Geometry check sheet. Reference: the model listing, model coordinates, mm. A direction names the side the tool comes from. Round coordinates to 2 decimals unless told otherwise and drop trailing zeros. Order: outer loops, then holes, each group sorted by start corner. A loop starts at its lowest first (then second) coordinate and runs counter-clockwise, first axis right, second up. Notation, with made-up numbers: (18, 58) - (32, 58) arc R21 ccw to (32, 75) - close; hole circle Ø10 at (21, 38). An arc over 180 degrees is marked (long way). One line per question, with ' | ' between items. Start each with the question number.
Q1. Sectioned sample at B-B, the plane z = -2. Give the number of separate pieces and of enclosed holes in the cut face, then the cut area to 3 significant figures.
Q2. Mould release check, pull along X, two halves, no side actions. Record for faces 3 (the face through (1, 12, -1)), 4 (the face through (-70.935, -5, -1)), 5 (the face through (41.515, 1.481, -1.369)): +X half, -X half, draft (parallel to the pull), parting line (faces both ways), or undercut.
Q3. Sectioned sample at C-C, the plane y = -5. Enter the section's corners in (x, z) (1 decimal), then the cut area to 3 significant figures.
Q4. Sectioned sample at A-A, the plane y = 1. Enter the section's corners in (x, z) (1 decimal), then the cut area to 3 significant figures.
Q5. Tool access check on faces 1 (the face through (-1, -23, -1)), 2 (the face through (63, 4, -1)). Record the directions out of +Z, -Z, +X, -X, +Y, -Y that give a thin tool (end or side, any length) a straight path to the whole face; none if there is none.
Q6. Material ranges on line 1 along X through (y, z) = (-4, -1.65) (1 decimal); line 2 along Y through (x, z) = (64, -1.75); line 3 along X through (y, z) = (-5.5, -2.5) (1 decimal), recorded low to high.
Solid Edge part; units mm, degrees
sketch "Sketch1" plane through (0, 0, 0) normal (0, 0, 1) x (1, 0, 0)
  line L0 (70.9315, 12) -> (-70.935, 12)
  line L1 (-70.935, 12) -> (-70.935, -23)
  line L2 (-70.935, -23) -> (70.9315, -23)
  line L3 (70.9315, -23) -> (70.9315, 12)
extrude "Protrusion1" add sketch "Sketch1" against normal blind 2.7
sketch "Sketch2" plane through (0, -5.5, -2.7) normal (0, 0, -1) x (-1, 0, 0)
  circle A0 centre (-49.2415, 12.5) radius 1.6
  circle A1 centre (-43.0415, 12.5) radius 1.6
  circle A2 centre (-49.2415, 6.5) radius 1.6
  circle A3 centre (-43.0415, 6.5) radius 1.6
  circle A4 centre (-49.2415, 0.5) radius 1.6
  circle A5 centre (-43.0415, 0.5) radius 1.6
  circle A6 centre (-49.2415, -5.5) radius 1.6
  circle A7 centre (-49.2415, -11.5) radius 1.6
  circle A8 centre (-43.0415, -5.5) radius 1.6
  circle A9 centre (-43.0415, -11.5) radius 1.6
extrude "Cutout1" cut sketch "Sketch2" against normal through all
mirror "Mirror1" about plane through (0, 0, 0) normal (1, 0, 0) of "Cutout1"
sketch "Sketch3" plane through (0, 0, 0) normal (0, 0, 1) x (1, 0, 0)
  line L0 (-64.935, 4) -> (-64.935, -1)
  line L1 (-64.935, -1) -> (-60.935, -1)
  line L2 (-60.935, -1) -> (-60.935, 4)
  line L3 (-60.935, 4) -> (-64.935, 4)
  line L4 (60.9315, -1) -> (64.9315, -1)
  line L5 (64.9315, -1) -> (64.9315, 4)
  line L6 (64.9315, 4) -> (60.9315, 4)
  line L7 (60.9315, 4) -> (60.9315, -1)
extrude "Cutout2" cut sketch "Sketch3" against normal up to next
properties material "MDF"
Determined:
1) separate pieces: 1 | enclosed holes: 22 | area: 4,760 mm2
2) face 3: draft | face 4: -X half | face 5: undercut
3) outline: (-70.9, -2.7) - (-50.8, -2.7) - (-50.8, 0) - (-70.9, 0) - close; (-47.6, -2.7) - (-44.6, -2.7) - (-44.6, 0) - (-47.6, 0) - close; (-41.4, -2.7) - (41.4, -2.7) - (41.4, 0) - (-41.4, 0) - close; (44.6, -2.7) - (47.6, -2.7) - (47.6, 0) - (44.6, 0) - close; (50.8, -2.7) - (70.9, -2.7) - (70.9, 0) - (50.8, 0) - close | area: 348 mm2
4) outline: (-70.9, -2.7) - (-64.9, -2.7) - (-64.9, 0) - (-70.9, 0) - close; (-60.9, -2.7) - (-50.8, -2.7) - (-50.8, 0) - (-60.9, 0) - close; (-47.6, -2.7) - (-44.6, -2.7) - (-44.6, 0) - (-47.6, 0) - close; (-41.4, -2.7) - (41.4, -2.7) - (41.4, 0) - (-41.4, 0) - close; (44.6, -2.7) - (47.6, -2.7) - (47.6, 0) - (44.6, 0) - close; (50.8, -2.7) - (60.9, -2.7) - (60.9, 0) - (50.8, 0) - close; (64.9, -2.7) - (70.9, -2.7) - (70.9, 0) - (64.9, 0) - close | area: 327 mm2
5) face 1: +Z, -Z, +X, -X, -Y | face 2: +Z, -Z
6) line 1: x = -70.9 to -50.5, -48 to -44.3, -41.8 to 41.8, 44.3 to 48, 50.5 to 70.9 | line 2: y = -23 to -1, 4 to 12 | line 3: x = -70.9 to -50.8, -47.7 to -44.6, -41.5 to 41.5, 44.6 to 47.7, 50.8 to 70.9
